Work out the finished part from the listing and answer in its coordinate system (mm). Coordinates: 2 decimals unless noted, no trailing zeros. Loops run counter-clockwise (first coordinate to the right, second up) from the corner with the lowest first, then second, coordinate; pieces in that order, holes last. Notation, with made-up numbers: (23.5, -32.5) - (31.5, -32.5) arc R22 ccw to (31.5, 0.5) - close; hole circle Ø1 at (79.5, -16.5). An arc over 180 degrees is marked (long way). Write each question's results on one line, items separated by ' | '. Start each with the question number.
Item 1: Section A-A, the plane x = 0 is taken. Write down the section's boundary in (y, z), plus the area to 3 significant figures.
Item 2: Section B-B, the plane z = 11.75 is taken. Write down the section's boundary in (x, y), plus the area to 3 significant figures.
Item 3: This flat-tipped pin is pushed along its axis until it touches: pin 1 Ø3.5 at (x, z) = (0, 16) entering from +Y. Where does it stop, or does it pass through?
Item 4: Consider probe 1 along Z at (x, y) = (0.25, 3); probe 2 along Z at (x, y) = (0.75, 2.75); probe 3 along X at (y, z) = (4.25, 16). Determine where each line is inside the solid, lowest interval first. Write a range as [from, to].
Item 5: For a pull along X with two mould halves and no side action, classify faces 1 (the face through (4.5, 6.5, 7.9)), 2 (the face through (0.1, 0.2, 20.2)), 3 (the face through (-2.685, 3.451, -0.596)) as +X half, -X half, draft (parallel to the pull), parting line (faces both ways), or undercut.
Item 6: Section C-C, the plane y = 2.25 is taken. Write down the section's boundary in (x, z), plus the area to 3 significant figures.
Item 7: Section D-D, the plane y = 6.25 is taken. Write down the section's boundary in (x, z).
from build123d import *

# Parameters (mm, degrees)
SKETCH_1_R      = 2.75
EXTRUDE_1_DEPTH = 7
CHAMFER_1_SIZE  = 1


with BuildPart() as part:
    # 草图1 → 凸台-拉伸1 (new body)
    with BuildSketch(Plane(origin=(0, 0, 0), x_dir=(1, 0, 0), z_dir=(0, 1, 0))):
        with BuildLine():
            Line((-5, -16), (-5, 0))
            ThreePointArc((-5, 0), (0, 5), (5, 0))
            Line((5, 0), (5, -16))
            ThreePointArc((5, -16), (0, -21), (-5, -16))
        make_face()
        with Locations(Location((0, 0, 0), (0, 0, 270))):
            Circle(SKETCH_1_R, mode=Mode.SUBTRACT)
        with Locations(Location((0, -16, 0), (0, 0, 270))):
            Circle(SKETCH_1_R, mode=Mode.SUBTRACT)
    extrude(amount=EXTRUDE_1_DEPTH)

    # 倒角1
    chamfer_1_edges = [part.edges().sort_by_distance(p)[0] for p in [
        (0, 7, -5),
        (-5, 7, 8),
        (0, 7, 21),
        (-5, 0, 8),
        (0, 0, -5),
        (5, 0, 8),
        (0, 0, 21),
        (5, 7, 8),
    ]]
    chamfer(chamfer_1_edges, length=CHAMFER_1_SIZE)


solid = part.part
Answer key:
1) outline: (0, -4) - (1, -5) - (6, -5) - (7, -4) - (7, -2.75) - (0, -2.75) - close; (0, 2.75) - (7, 2.75) - (7, 13.25) - (0, 13.25) - close; (0, 18.75) - (7, 18.75) - (7, 20) - (6, 21) - (1, 21) - (0, 20) - close | area: 103 mm^2
2) outline: (-5, 1) - (-4, 0) - (4, 0) - (5, 1) - (5, 6) - (4, 7) - (-4, 7) - (-5, 6) - close | area: 68.0 mm^2
3) pin 1: passes through
4) probe 1: z = [-4.99, -2.74], [2.74, 13.26], [18.74, 20.99] | probe 2: z = [-4.94, -2.65], [2.65, 13.35], [18.65, 20.94] | probe 3: x = [-5, -2.75], [2.75, 5]
5) face 1: +X half | face 2: parting line | face 3: undercut
6) outline: (-5, 0) arc R5 ccw to (5, 0) - (5, 16) arc R5 ccw to (-5, 16) - close; hole circle Ø5.5 at (0, 0); hole circle Ø5.5 at (0, 16) | area: 191 mm^2
7) outline: (-4.75, 0) arc R4.75 ccw to (4.75, 0) - (4.75, 16) arc R4.75 ccw to (-4.75, 16) - close; hole circle Ø5.5 at (0, 0); hole circle Ø5.5 at (0, 16)
